The model under review builds one solid part; all positions refer to its coordinate system, in mm. A direction names the side the tool comes from. Coordinates: 2 decimals unless noted, no trailing zeros. Write item = value, one per line. Start each with the question number.
Q1. Wall thickness on probe 1 along X at (y, z) = (0.25, -44) (3 decimals); probe 2 along Z at (x, y) = (49.57, 1.2); probe 3 along Z at (x, y) = (49, 1.6): over which ranges is each line inside the solid? List them lowest first.
Q2. We need section A-A on x = 49.57. Count the separate pieces of the cut face and the enclosed holes in it, and give its area (3 significant figures).
Q3. For faces 1 (the face through (-53.445, 2, 44)), 2 (the face through (68.745, 2, 1)), list the 3-axis set-ups (+Z, -Z, +X, -X, +Y, -Y) from which the entire face can be reached by the end or side of a thin tool; tool diameter is ignored.
Q4. Clearance check with a flat-ended pin moving along its axis: pin 1 Ø2.5 at (x, z) = (49.57, 44.17) entering from +Y. State where the tip first meets the part, or that it passes through.
Q5. Mouldability with a two-part tool opening along Z and no side actions: class faces 3 (the face through (-1, 2, 48.172)), 4 (the face through (59, 2, -42.426)), 5 (the face through (-1, 0, -1)) as released by +Z, released by -Z, zero draft, split by the parting line, or undercut.
from build123d import *

# Parameters (mm, degrees)
SKETCH1_W                                      = 137.49
SKETCH1_H                                      = 96.345
SKETCH1_R                                      = 2.5
SKETCH1_W_2                                    = 10.25
SKETCH1_H_2                                    = 3.4925
BOSS_EXTRUDE1_DEPTH                            = 3.175
CUT_EXTRUDE1_START                             = -1
SKETCH1_3_W                                    = 10.25
SKETCH1_3_H                                    = 3.4925
CUT_EXTRUDE1_DEPTH                             = 5.175
M2_5_CLEARANCE_HOLE1_D                         = 2.9
M2_5_CLEARANCE_HOLE1_CSINK_D                   = 2.95
M2_5_CLEARANCE_HOLE1_CSINK_ANGLE               = 100
MIRROR1_START                                  = -1
MIRROR1_AT_THE_SECOND_PLANE_COPY_1_SKETC_W     = 10.25
MIRROR1_AT_THE_SECOND_PLANE_COPY_1_SKETC_H     = 3.4925
MIRROR1_AT_THE_SECOND_PLANE_COPY_1_DEPTH       = 5.175
MIRROR1_AT_THE_SECOND_PLANE_COPY_2_D           = 2.9
MIRROR1_AT_THE_SECOND_PLANE_COPY_2_CSINK_D     = 2.95
MIRROR1_AT_THE_SECOND_PLANE_COPY_2_CSINK_ANGLE = 100
FILLET1_R                                      = 1


with BuildPart() as part:
    # Sketch1 → Boss-Extrude1 (new body)
    with BuildSketch(Plane(origin=(0, 0, 0), x_dir=(1, 0, 0), z_dir=(0, 1, 0))):
        Rectangle(SKETCH1_W, SKETCH1_H)
        with Locations((-49.57, 44.1725)):
            Circle(SKETCH1_R, mode=Mode.SUBTRACT)
        with Locations((-58.57, 44.1725)):
            Rectangle(SKETCH1_W_2, SKETCH1_H_2, mode=Mode.SUBTRACT)
        with Locations((-58.57, 44.1725)):
            Rectangle(SKETCH1_W_2, SKETCH1_H_2)
        with Locations((-49.57, 44.1725)):
            Circle(SKETCH1_R)
    extrude(amount=BOSS_EXTRUDE1_DEPTH)

    # Sketch1<3> → Cut-Extrude1 (cut)
    with BuildSketch(Plane(origin=(0, 0, 0), x_dir=(1, 0, 0), z_dir=(0, 1, 0)).offset(CUT_EXTRUDE1_START)):
        with Locations((-58.57, 44.1725)):
            Rectangle(SKETCH1_3_W, SKETCH1_3_H)
    cut_extrude1 = extrude(amount=CUT_EXTRUDE1_DEPTH, mode=Mode.SUBTRACT)

    # M2.5 Clearance Hole1 (through all)
    with Locations(Plane(origin=(0, 3.175, 0), x_dir=(1, 0, 0), z_dir=(0, 1, 0))):
        with Locations((-49.57, 44.1725)):
            m2_5_clearance_hole1 = CounterSinkHole(M2_5_CLEARANCE_HOLE1_D / 2, M2_5_CLEARANCE_HOLE1_CSINK_D / 2, counter_sink_angle=M2_5_CLEARANCE_HOLE1_CSINK_ANGLE)

    # Mirror1: Cut-Extrude1, M2.5 Clearance Hole1 across plane
    add(cut_extrude1.mirror(Plane(origin=(0, 0, 0), x_dir=(0, 0, 1), z_dir=(1, 0, 0))), mode=Mode.SUBTRACT)
    add(m2_5_clearance_hole1.mirror(Plane(origin=(0, 0, 0), x_dir=(0, 0, 1), z_dir=(1, 0, 0))), mode=Mode.SUBTRACT)

    # Mirror1 at the second plane: M2.5 Clearance Hole1, Cut-Extrude1 across plane
    add(m2_5_clearance_hole1.mirror(Plane.XY), mode=Mode.SUBTRACT)
    add(cut_extrude1.mirror(Plane.XY), mode=Mode.SUBTRACT)

    # Mirror1 at the second plane copy 1 sketc → Mirror1 at the second plane copy 1 (cut)
    with BuildSketch(Plane(origin=(0, 0, 0), x_dir=(-1, 0, 0), z_dir=(0, 1, 0)).offset(MIRROR1_START)):
        with Locations((-58.57, 44.1725)):
            Rectangle(MIRROR1_AT_THE_SECOND_PLANE_COPY_1_SKETC_W, MIRROR1_AT_THE_SECOND_PLANE_COPY_1_SKETC_H)
    extrude(amount=MIRROR1_AT_THE_SECOND_PLANE_COPY_1_DEPTH, mode=Mode.SUBTRACT)

    # Mirror1 at the second plane copy 2 (through all)
    with Locations(Plane(origin=(0, 3.175, 0), x_dir=(-1, 0, 0), z_dir=(0, 1, 0))):
        with Locations((-49.57, 44.1725)):
            CounterSinkHole(MIRROR1_AT_THE_SECOND_PLANE_COPY_2_D / 2, MIRROR1_AT_THE_SECOND_PLANE_COPY_2_CSINK_D / 2, counter_sink_angle=MIRROR1_AT_THE_SECOND_PLANE_COPY_2_CSINK_ANGLE)

    # Fillet1
    fillet1_edges = [part.edges().sort_by_distance(p)[0] for p in [
        (-68.745, 1.5875, 48.1725),
        (-68.745, 1.5875, -48.1725),
        (68.745, 1.5875, -48.1725),
        (68.745, 1.5875, 48.1725),
    ]]
    fillet(fillet1_edges, radius=FILLET1_R)


solid = part.part
Returned:
q1.probe_1 = -68.745 to -63.695, -53.445 to -51.01, -48.13 to 48.13, 51.01 to 53.445, 63.695 to 68.745
q1.probe_2 = -48.17 to -45.62, -42.72 to 42.72, 45.62 to 48.17
q1.probe_3 = -48.17 to -45.51, -42.84 to 42.84, 45.51 to 48.17
q2.separate_pieces = 3
q2.enclosed_holes = 0
q2.area = 287 mm^2
q3.face_1 = +Y, -Y
q3.face_2 = +Z, -Z, +X, +Y, -Y
q4.pin_1 = through
q5.face_3 = released by +Z
q5.face_4 = undercut
q5.face_5 = zero draft
